Verification items for the finished model (mm, model axes). Face numbers are marked on the shaded views. A direction names the side the tool comes from. Coordinates: 2 decimals unless noted, no trailing zeros. Order: outer loops, then holes, each group sorted by start corner. A loop starts at its lowest first (then second) coordinate and runs counter-clockwise, first axis right, second up. Notation, with made-up numbers: (60, 73) - (98, 73) arc R15 ccw to (98, 90) - close; hole circle Ø10 at (-13, 61.5). An arc over 180 degrees is marked (long way). Answer as CSV lines item,"result". Start each with the question number.
1. Set-up check for the marked faces 4 and 5: record each of +Z, -Z, +X, -X, +Y, -Y from which the full face is reachable in a straight line by a thin tool's end or side.
2. Mould release check, pull along Z, two halves, no side actions. Record for the marked faces 1, 2 and 3: pulls with the +Z half, pulls with the -Z half, needs draft (parallel to the pull), parting line crosses it, or undercut.
3. Material ranges on L1, parallel to Z at x = -0.5, y = -6.5; L2, parallel to X at y = -2, z = 93; L3, parallel to Z at x = -3, y = 4.25, recorded low to high. Write a range as [from, to].
4. Section check A-A (z = 0). Record the cut outline in (x, y).
5. Section check B-B (x = 2). Record the cut outline in (y, z), and give its area (3 significant figures).
6. Section check C-C (y = -6.5). Count the separate pieces of the cut face and the enclosed holes in it, and give its area (3 significant figures).
7. Go/stop test with flat-tipped pins: pin 1 (1 mm diameter, centred on x = -11.5, y = 5.5, fed in from -Z); pin 2 (5.5 mm diameter, centred on x = 16.27, y = 0, fed in from +Z); pin 3 (3 mm diameter, centred on x = -15, y = 3.5, fed in from +Z); pin 4 (5 mm diameter, centred on y = -1, z = 53.5, fed in from +X). Record where each tip stops, or that it passes through.
from build123d import *

# Parameters (mm, degrees)
F0_R        = 7.1501
F0_R_2      = 10.95375
F1_DEPTH    = 7.9121
F2_T1_DEPTH = 64.0588
F3_R        = 3.34264
F4_DEPTH    = 103.5501653159


# Not quite as in the source:
# - a fillet or chamfer that OpenCascade refuses, or shapes differently, is made with other operations: its cross-section is extruded or revolved along the edge and cut away or added
# - a feature names something its author has since deleted; it is built from what else it names


with BuildPart() as f1:
    # F0 (on Front) → F1 (new body, symmetric)
    with BuildSketch(Plane.XZ):
        with BuildLine():
            ThreePointArc((-10.9740144438, 76.3394153159), (-10.3105393191, 75.7356011824), (-9.6139, 75.1703716645))
            Line((-9.6139, 75.1703716645), (-6.604, 8.5633440549))
            ThreePointArc((-6.604, 8.5633440549), (0, -10.81405), (6.604, 8.5633440549))
            Line((6.604, 8.5633440549), (9.6139, 75.1703716645))
            ThreePointArc((9.6139, 75.1703716645), (10.3105393191, 75.7356011824), (10.9740144438, 76.3394153159))
            Line((10.9740144438, 76.3394153159), (21.57095, 76.3394153159))
            Line((21.57095, 76.3394153159), (21.57095, 99.1232153159))
            Line((21.57095, 99.1232153159), (10.9740144438, 99.1232153159))
            ThreePointArc((10.9740144438, 99.1232153159), (0, 103.5491653159), (-10.9740144438, 99.1232153159))
            Line((-10.9740144438, 99.1232153159), (-21.57095, 99.1232153159))
            Line((-21.57095, 99.1232153159), (-21.57095, 76.3394153159))
            Line((-21.57095, 76.3394153159), (-10.9740144438, 76.3394153159))
        make_face()
        Circle(F0_R, mode=Mode.SUBTRACT)
        with Locations((0, 87.7313153159)):
            Circle(F0_R_2, mode=Mode.SUBTRACT)
    extrude(amount=F1_DEPTH, both=True)

    # F2: fillet of radius 8.255 on 4 edges, made by hand

    # F2_s2 → F2_t1 (cut)
    with BuildSketch(Plane.XY.offset(55.7019153159)):
        with BuildLine():
            add(Edge.make_bspline(
                [(-13.31595, -7.9121), (-21.57095, -7.9121), (-21.57095, 0.3429)],
                knots=[0, 0, 0, 1, 1, 1], degree=2, weights=[1, 1, 1]))
            Line((-21.57095, 0.3429), (-21.57095, -7.9121))
            Line((-21.57095, -7.9121), (-13.31595, -7.9121))
        make_face()
        with BuildLine():
            add(Edge.make_bspline(
                [(-21.57095, -0.3429), (-21.57095, 7.9121), (-13.31595, 7.9121)],
                knots=[0, 0, 0, 1, 1, 1], degree=2, weights=[1, 1, 1]))
            Line((-13.31595, 7.9121), (-21.57095, 7.9121))
            Line((-21.57095, 7.9121), (-21.57095, -0.3429))
        make_face()
        with BuildLine():
            add(Edge.make_bspline(
                [(21.57095, 0.3429), (21.57095, -7.9121), (13.31595, -7.9121)],
                knots=[0, 0, 0, 1, 1, 1], degree=2, weights=[1, 1, 1]))
            Line((13.31595, -7.9121), (21.57095, -7.9121))
            Line((21.57095, -7.9121), (21.57095, 0.3429))
        make_face()
        with BuildLine():
            add(Edge.make_bspline(
                [(21.57095, -0.3429), (21.57095, 7.9121), (13.31595, 7.9121)],
                knots=[0, 0, 0, 1, 1, 1], degree=2, weights=[1, 1, 1]))
            Line((13.31595, 7.9121), (21.57095, 7.9121))
            Line((21.57095, 7.9121), (21.57095, -0.3429))
        make_face()
    extrude(amount=F2_T1_DEPTH, mode=Mode.SUBTRACT)

    # F3 (on Top) → F4 (cut, through all)
    with BuildSketch(Plane.XY):
        with Locations((-16.2724846, 0)):
            Circle(F3_R)
        with Locations((16.2724877468, 0)):
            Circle(F3_R)
    extrude(amount=F4_DEPTH, mode=Mode.SUBTRACT)


solid = f1.part
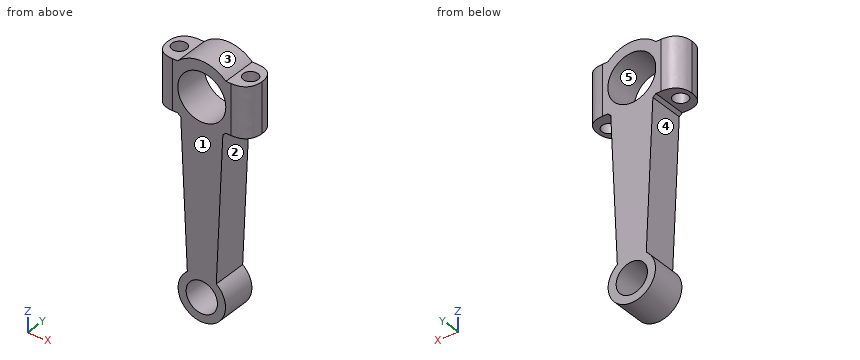
Evaluation:
1,face 4,"-X, +Y, -Y"
1,face 5,"+Y, -Y"
2,face 1,"needs draft"
2,face 2,"undercut"
2,face 3,"pulls with the +Z half"
3,L1,"z = [-10.8, -7.13], [7.13, 76.79], [98.67, 103.54]"
3,L2,"x = [-21.38, -18.95], [-13.59, -9.6], [9.6, 13.59], [18.95, 21.38]"
3,L3,"z = [-10.39, -6.49], [6.49, 77.2], [98.27, 103.26]"
4,outline,"(-10.81, -7.91) - (-7.15, -7.91) - (-7.15, 7.91) - (-10.81, 7.91) - close; (7.15, -7.91) - (10.81, -7.91) - (10.81, 7.91) - (7.15, 7.91) - close"
5,outline,"(-7.91, -10.63) - (7.91, -10.63) - (7.91, -6.86) - (-7.91, -6.86) - close; (-7.91, 6.86) - (7.91, 6.86) - (7.91, 76.96) - (-7.91, 76.96) - close; (-7.91, 98.5) - (7.91, 98.5) - (7.91, 103.42) - (-7.91, 103.42) - close"
5,area,"1,250 mm²"
6,separate pieces,"1"
6,enclosed holes,"2"
6,area,"1,830 mm²"
7,pin 1,"stops at z = 76.34"
7,pin 2,"passes through"
7,pin 3,"stops at z = 99.12"
7,pin 4,"stops at x = 8.75"
